Geometry check sheet. Reference: drawing and pictorial views, mm from the part's lowest x, y, z. A direction names the side the tool comes from. Give positions to 0.01 mm unless a question says otherwise; leave off trailing zeros. Loops run counter-clockwise (first coordinate to the right, second up) from the corner with the lowest first, then second, coordinate; pieces in that order, holes last. Notation, with made-up numbers: (-2.75, 85.25) - (48.25, 85.25) arc R17 ccw to (48.25, 109.25) - close; hole circle Ø1 at (-28, 55.25). An arc over 180 degrees is marked (long way). Answer in a Markdown table with one row per item. Add a question column.
(1) Sectioned sample at A-A on y = 1.6. Enter the section's corners in (x, z).
(2) Sectioned sample at D-D on x = 10. Enter the section's corners in (y, z).
(3) Go/stop test with a flat-tipped pin: P1, Ø1, axis at y = 1, z = 1, coming from the +X side. Record where the tip stops, or that it passes through.
(4) Thickness scan on L1, parallel to X at y = 2.8, z = 1.7; L2, parallel to Z at x = 2.5, y = 2.85. Record the ranges inside material, lowest first.
(5) Set-up check for the marked faces 1 and 2: record each of +Z, -Z, +X, -X, +Y, -Y from which the full face is reachable in a straight line by a thin tool's end or side.
(6) Sectioned sample at C-C on y = 0.2. Enter the section's corners in (x, z).
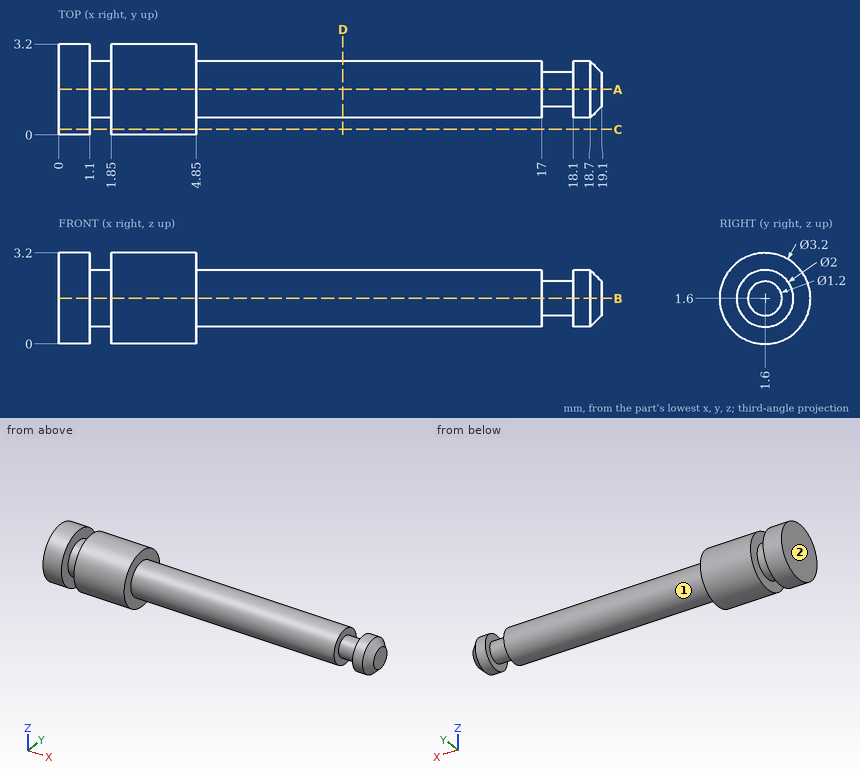
Reply:
| question | item | result |
|---|---|---|
| 1 | outline | (0, 0) - (1.1, 0) - (1.1, 0.6) - (1.85, 0.6) - (1.85, 0) - (4.85, 0) - (4.85, 0.6) - (17, 0.6) - (17, 1) - (18.1, 1) - (18.1, 0.6) - (18.7, 0.6) - (19.1, 1) - (19.1, 2.2) - (18.7, 2.6) - (18.1, 2.6) - (18.1, 2.2) - (17, 2.2) - (17, 2.6) - (4.85, 2.6) - (4.85, 3.2) - (1.85, 3.2) - (1.85, 2.6) - (1.1, 2.6) - (1.1, 3.2) - (0, 3.2) - close |
| 2 | outline | circle Ø2 at (1.6, 1.6) |
| 3 | P1 | x = 19.1 |
| 4 | L1 | 0 to 1.1, 1.85 to 4.85 |
| 4 | L2 | 0.6 to 2.6 |
| 5 | face 1 | +X |
| 5 | face 2 | +Z, -Z, -X, +Y, -Y |
| 6 | outline | (0, 0.83) - (1.1, 0.83) - (1.1, 2.37) - (0, 2.37) - close; (1.85, 0.83) - (4.85, 0.83) - (4.85, 2.37) - (1.85, 2.37) - close |
